Answer from the drawing. Dimensions are ordinates in mm from the lowest x, y and z of the part. A direction names the side the tool comes from. Coordinates: 2 decimals unless noted, no trailing zeros. Order: outer loops, then holes, each group sorted by start corner. A loop starts at its lowest first (then second) coordinate and runs counter-clockwise, first axis right, second up. Notation, with made-up numbers: M 22.25,15.5 L 67.25,15.5 A22 ccw 67.25,33.5 Z; hole C -23,6.25 d2. An arc over 180 degrees is marked long. Use a Markdown table: item, result.
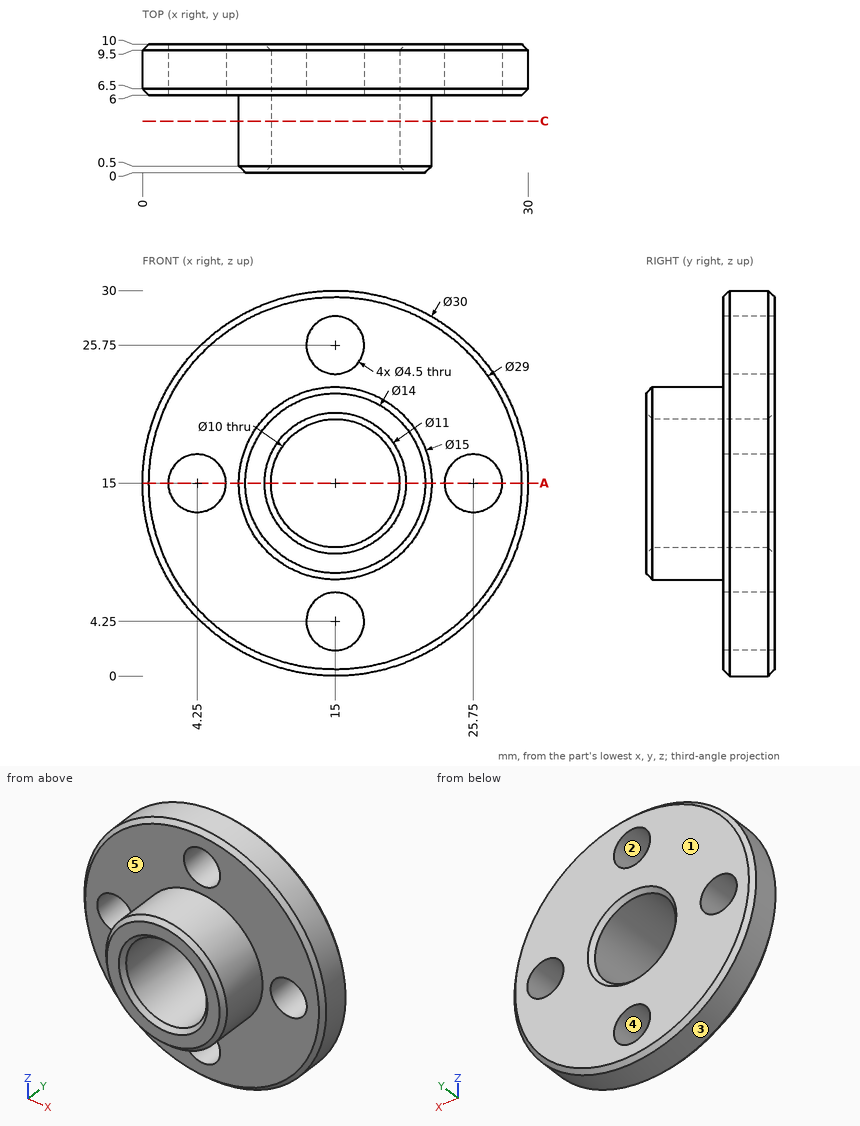
(1) A cutting plane is placed at A-A (z = 15). Give the number of separate pieces and of enclosed holes in the cut face, then the cut area to 4 significant figures.
Conclusion:
| item | result |
|---|---|
| separate pieces | 4 |
| enclosed holes | 0 |
| area | 72.75 mm2 |
(2) Determine the mould class of the marked faces 1, 2 and 3 for opening direction X: pulls with the +X half, pulls with the -X half, needs draft (parallel to the pull), parting line crosses it, or undercut.
Conclusion:
| item | result |
|---|---|
| face 1 | needs draft |
| face 2 | undercut |
| face 3 | parting line crosses it |
(3) A cutting plane is placed at C-C (y = 4). Determine the outline of the cut face in (x, z), then the cut area to 3 significant figures.
Conclusion:
| item | result |
|---|---|
| outline | C 15,15 d15; hole C 15,15 d10 |
| area | 98.2 mm2 |
(4) Given P1, Ø4, axis at x = 6, z = 7, coming from the -Y side; P2, Ø2, axis at y = 3.5, z = 14, coming from the -X side; P3, Ø7, axis at x = 4.25, z = 15, coming from the -Y side; P4, Ø3.5, axis at x = 15, z = 4.25, coming from the -Y side, each flat-ended and moving along its own axis, determine where each tip first touches the part or whether it passes through.
Conclusion:
| item | result |
|---|---|
| P1 | y = 6 |
| P2 | x = 7.5 |
| P3 | y = 0.25 |
| P4 | through |
(5) Which of the six approach directions +Z, -Z, +X, -X, +Y, -Y give full straight-line access (tool end or side, diameter ignored) to the marked faces 4 and 5?
Conclusion:
| item | result |
|---|---|
| face 4 | +Y, -Y |
| face 5 | -Y |
(6) Straight lines are drawn through the part: L1, parallel to Z at x = 15, y = 7.25; L2, parallel to X at y = 6.25, z = 16.25; L3, parallel to Z at x = 15, y = 4. For each, find the intervals that lie inside material, in ascending order.
Conclusion:
| item | result |
|---|---|
| L1 | 0 to 2, 6.5 to 10, 20 to 23.5, 28 to 30 |
| L2 | 0.3 to 2.38, 6.12 to 10.16, 19.84 to 23.88, 27.62 to 29.7 |
| L3 | 7.5 to 10, 20 to 22.5 |
